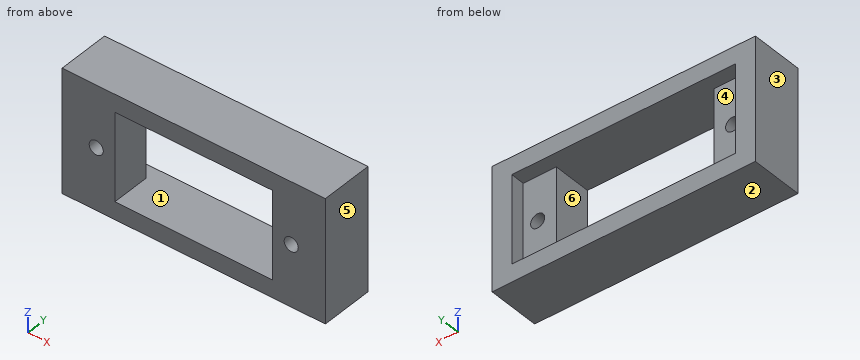
```python
from build123d import *

# Parameters (mm, degrees)
SKETCH1_W           = 37.4
SKETCH1_H           = 17.5
SKETCH1_R           = 1
SKETCH1_W_2         = 22.4
SKETCH1_H_2         = 12.5
BOSS_EXTRUDE1_DEPTH = 7.46
SKETCH2_W           = 31.8
SKETCH2_H           = 12.5
CUT_EXTRUDE1_DEPTH  = 2


with BuildPart() as part:
    # Sketch1 → Boss-Extrude1 (new body)
    with BuildSketch(Plane(origin=(0, 0, 0), x_dir=(1, 0, 0), z_dir=(0, 1, 0))):
        Rectangle(SKETCH1_W, SKETCH1_H)
        with Locations(Location((13.85, 0, 0), (0, 0, 270))):
            Circle(SKETCH1_R, mode=Mode.SUBTRACT)
        with Locations(Location((-13.85, 0, 0), (0, 0, 270))):
            Circle(SKETCH1_R, mode=Mode.SUBTRACT)
        Rectangle(SKETCH1_W_2, SKETCH1_H_2, mode=Mode.SUBTRACT)
    extrude(amount=-BOSS_EXTRUDE1_DEPTH)

    # Sketch2 → Cut-Extrude1 (cut)
    with BuildSketch(Plane(origin=(0, 0, 0), x_dir=(1, 0, 0), z_dir=(0, 1, 0))):
        Rectangle(SKETCH2_W, SKETCH2_H)
    extrude(amount=-CUT_EXTRUDE1_DEPTH, mode=Mode.SUBTRACT)


solid = part.part
```
Read the model definition and answer for the solid it produces. Units are mm, in the model's axes. Face numbers are marked on the shaded views. A direction names the side the tool comes from. Give positions to 0.01 mm unless a question says otherwise; leave off trailing zeros. Write each loop counter-clockwise with the first axis right and the second up, starting at its lowest first coordinate (ties: lowest second). Pieces come first, ordered by that corner, then holes. Notation, with made-up numbers: (-11, 42.25) -> (41, 42.25) arc R17 cw to (41, 46.25) -> close; hole circle Ø10 at (60, 60). An arc over 180 degrees is marked (long way). Answer as a JSON object with one key per item and string values.
1) Straight lines are drawn through the part: probe 1 along X at (y, z) = (-3.9, 0); probe 2 along X at (y, z) = (-5, -1.75); probe 3 along Z at (x, y) = (7, -1.5). For each, find the intervals that lie inside material, in ascending order. Write a range as from..to.
Findings below:
{"probe 1": "x = -18.7..-14.85, -12.85..-11.2, 11.2..12.85, 14.85..18.7", "probe 2": "x = -18.7..-11.2, 11.2..18.7", "probe 3": "z = -8.75..-6.25, 6.25..8.75"}
2) For a pull along Z with two mould halves and no side action, classify the marked faces 1, 2 and 3 as pulls with the +Z half, pulls with the -Z half, needs draft (parallel to the pull), parting line crosses it, or undercut.
Findings below:
{"face 1": "undercut", "face 2": "pulls with the -Z half", "face 3": "needs draft"}
3) A flat-ended cylindrical pin translates along its axis: pin 1 Ø2.5 at (x, z) = (13.85, 0) entering from +Y. Find the tip coordinate at first contact, or state that the pin passes through.
Findings below:
{"pin 1": "stops at y = -2"}
4) Section D-D on z = 0 is taken. Write down the section's boundary in (x, y).
Findings below:
{"outline": "(-18.7, -7.46) -> (-14.85, -7.46) -> (-14.85, -2) -> (-15.9, -2) -> (-15.9, 0) -> (-18.7, 0) -> close; (-12.85, -7.46) -> (-11.2, -7.46) -> (-11.2, -2) -> (-12.85, -2) -> close; (11.2, -7.46) -> (12.85, -7.46) -> (12.85, -2) -> (11.2, -2) -> close; (14.85, -7.46) -> (18.7, -7.46) -> (18.7, 0) -> (15.9, 0) -> (15.9, -2) -> (14.85, -2) -> close"}
5) A tool of negligible diameter and unlimited length cuts with its end or side. For the marked faces 4, 5 and 6, from which of +Z, -Z, +X, -X, +Y, -Y can it reach the whole face along a straight path? Write none if from no direction.
Findings below:
{"face 4": "+Y", "face 5": "+Z, -Z, +X, +Y, -Y", "face 6": "+Y, -Y"}
6) Section A-A on z = -4 is taken. Write down the section's boundary in (x, y).
Findings below:
{"outline": "(-18.7, -7.46) -> (-11.2, -7.46) -> (-11.2, -2) -> (-15.9, -2) -> (-15.9, 0) -> (-18.7, 0) -> close; (11.2, -7.46) -> (18.7, -7.46) -> (18.7, 0) -> (15.9, 0) -> (15.9, -2) -> (11.2, -2) -> close"}
7) Section B-B on x = 9 is taken. Write down the section's boundary in (y, z).
Findings below:
{"outline": "(-7.46, -8.75) -> (0, -8.75) -> (0, -6.25) -> (-7.46, -6.25) -> close; (-7.46, 6.25) -> (0, 6.25) -> (0, 8.75) -> (-7.46, 8.75) -> close"}
8) Section C-C on y = -1 is taken. Write down the section's boundary in (x, z).
Findings below:
{"outline": "(-18.7, -8.75) -> (18.7, -8.75) -> (18.7, 8.75) -> (-18.7, 8.75) -> close; hole (-15.9, -6.25) -> (15.9, -6.25) -> (15.9, 6.25) -> (-15.9, 6.25) -> close"}
